Autodesk Inventor part; units mm, degrees
ref_plane "YZ Plane" through (0, 0, 0) normal (1, 0, 0) x (0, 1, 0)
ref_plane "XZ Plane" through (0, 0, 0) normal (0, 1, 0) x (-1, 0, 0)
ref_plane "XY Plane" through (0, 0, 0) normal (0, 0, 1) x (1, 0, 0)
sketch "スケッチ1" plane through (0, 0, 0) normal (0, 1, 0) x (-1, 0, 0)
  line L0 (0, 0) -> (-21, 0)
  line L1 (-21, 0) -> (-21, -7.5)
  line L2 (-21, -7.5) -> (0, -7.5)
  line L3 (0, -7.5) -> (0, 0)
  dimension "d1" = 21
  dimension "d27" = 7.5
extrude "押し出し1" add sketch "スケッチ1" along normal blind 2
sketch "スケッチ2" plane through (0, 2, 0) normal (0, 1, 0) x (1, 0, 0)
  line L0 (0, 7.5) -> (0, 0)
  line L1 (0, 3.75) -> (21, 3.75)
  line L2 (21, 0) -> (21, 7.5)
  line L3 (0, 0) -> (21, 0)
  line L4 (10.5, 0) -> (10.5, 7.5)
  line L5 (21, 7.5) -> (0, 7.5)
  line L6 (4, 0) -> (4, 7.5)
  line L7 (17, 0) -> (17, 7.5)
  point P0 (4, 3.75)
  point P1 (17, 3.75)
  dimension "d18" = 3.75
  dimension "d19" = 3.75
  dimension "d20" = 21
  dimension "d23" = 4
  dimension "d24" = 4
hole "穴1" at (4, 2, -3.75) at (17, 2, -3.75) direction (0, -1, 0) diameter 4.5 end through all
fillet "フィレット1" radius 3.5 4 edges at (21, 1, 0) (21, 1, -7.5) (0, 1, 0) (0, 1, -7.5)
properties part number "Plate" material "鋼、軟鋼"
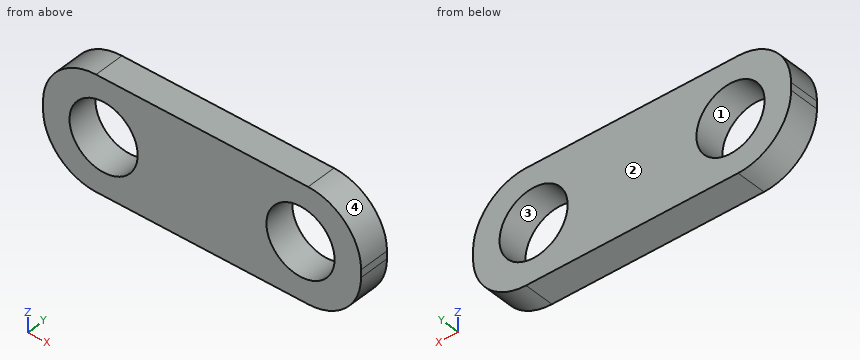
Check sheet for the modelled part. Datum: model origin and axes. Units: mm. Face numbers are marked on the shaded views. Give positions to 0.01 mm unless a question says otherwise; leave off trailing zeros. Loops run counter-clockwise (first coordinate to the right, second up) from the corner with the lowest first, then second, coordinate; pieces in that order, holes last. Notation, with made-up numbers: M 29,47.25 L 83,47.25 A24 ccw 83,78.25 Z; hole C 70.5,-7.5 d2. An arc over 180 degrees is marked long. Answer as a JSON object with one key per item and string values. Group by question number.
Q1. Release check for a two-part mould opening along X. For the marked faces 1, 2, 3 and 4 record: released by +X, released by -X, zero draft, split by the parting line, or undercut.
Q2. Cross-section at A-A on x = 4. Record the cut outline in (y, z), then the cut area to 3 significant figures.
Q3. Cross-section at C-C on y = 0.3. Record the cut outline in (x, z), then the cut area to 3 significant figures.
Q4. Cross-section at D-D on x = 19.75. Record the cut outline in (y, z).
Q5. Cross-section at B-B on z = -3.75. Record the cut outline in (x, y).
Q6. Material ranges on line 1 along X through (y, z) = (0.9, -3.75); line 2 along Z through (x, y) = (4, 0.75); line 3 along X through (y, z) = (1.6, -2.25), recorded low to high. Write a range as [from, to].
Evaluation:
{
 "1": {"face 1": "undercut", "face 2": "zero draft", "face 3": "undercut", "face 4": "released by +X"},
 "2": {"outline": "M 0,-7.5 L 2,-7.5 L 2,-6 L 0,-6 Z; M 0,-1.5 L 2,-1.5 L 2,0 L 0,0 Z", "area": "6.00 mm2"},
 "3": {"outline": "M 0,-4 A3.5 ccw 3.5,-7.5 L 17.5,-7.5 A3.5 ccw 21,-4 L 21,-3.5 A3.5 ccw 17.5,0 L 3.5,0 A3.5 ccw 0,-3.5 Z; hole C 4,-3.75 d4.5; hole C 17,-3.75 d4.5", "area": "115 mm2"},
 "4": {"outline": "M 0,-6.68 L 2,-6.68 L 2,-0.82 L 0,-0.82 Z"},
 "5": {"outline": "M 0,0 L 1.75,0 L 1.75,2 L 0,2 Z; M 6.25,0 L 14.75,0 L 14.75,2 L 6.25,2 Z; M 19.25,0 L 21,0 L 21,2 L 19.25,2 Z"},
 "6": {"line 1": "x = [0, 1.75], [6.25, 14.75], [19.25, 21]", "line 2": "z = [-7.5, -6], [-1.5, 0]", "line 3": "x = [0.23, 2.32], [5.68, 15.32], [18.68, 20.77]"}
}
